```python
from build123d import *

# Parameters (mm, degrees)
SKETCH1_W                = 45
SKETCH1_H                = 40
BOSS_EXTRUDE1_DEPTH      = 50
SKETCH2_W                = 15
SKETCH2_H                = 10
CUT_EXTRUDE1_DEPTH       = 68.869359802
SKETCH6_W                = 20
SKETCH6_H                = 30
CUT_EXTRUDE15_DEPTH      = 33
CUT_EXTRUDE16_DEPTH      = 59.36308765
CUT_EXTRUDE16_DEPTH_BACK = 20


with BuildPart() as part:
    # Sketch1 → Boss-Extrude1 (new body)
    with BuildSketch(Plane(origin=(0, 0, 0), x_dir=(1, 0, 0), z_dir=(0, 1, 0))):
        Rectangle(SKETCH1_W, SKETCH1_H)
    extrude(amount=BOSS_EXTRUDE1_DEPTH)

    # Sketch2 → Cut-Extrude1 (cut, through all)
    with BuildSketch(Plane.XY.offset(20)):
        with Locations((0, 5)):
            Rectangle(SKETCH2_W, SKETCH2_H)
    extrude(amount=-CUT_EXTRUDE1_DEPTH, mode=Mode.SUBTRACT)

    # Sketch6 → Cut-Extrude15 (cut)
    with BuildSketch(Plane.ZY.offset(22.5)):
        with Locations((10, 35)):
            Rectangle(SKETCH6_W, SKETCH6_H)
    extrude(amount=-CUT_EXTRUDE15_DEPTH, mode=Mode.SUBTRACT)

    # Sketch7 → Cut-Extrude16 (cut, two sides: drawn at the far end of the back side and taken through both)
    with BuildSketch(Plane.XY.offset(-CUT_EXTRUDE16_DEPTH_BACK)):
        Polygon((106.556450077, 137.324045524), (10.5, 50), (-22.5, 20), (-118.556450077, -67.324045524), (-293.204541126, 124.788854629), (-68.091640972, 329.436945678), align=None)
    extrude(amount=CUT_EXTRUDE16_DEPTH + CUT_EXTRUDE16_DEPTH_BACK, mode=Mode.SUBTRACT)


solid = part.part
```
Geometry check sheet. Reference: the model listing, model coordinates, mm. A direction names the side the tool comes from. Coordinates: 2 decimals unless noted, no trailing zeros. Write each loop counter-clockwise with the first axis right and the second up, starting at its lowest first coordinate (ties: lowest second). Pieces come first, ordered by that corner, then holes. Notation, with made-up numbers: (-35, -33) -> (-13, -33) arc R21 ccw to (-13, 0) -> close; hole circle Ø11 at (-38.75, -23). An arc over 180 degrees is marked (long way). Use CSV: the item, a comma, the result in double quotes. Start each with the question number.
Item 1: Cross-section at A-A, the plane z = -10.5. Record the cut outline in (x, y), plus the area to 4 significant figures.
Item 2: Cross-section at B-B, the plane y = 39.5. Record the cut outline in (x, z), plus the area to 3 significant figures.
Item 3: Depth check by flat-ended pin: pin 1 Ø9 at (x, y) = (-11, 33) entering from +Z; pin 2 Ø2 at (x, z) = (-1.5, -9) entering from -Y; pin 3 Ø4 at (y, z) = (29.5, 13.5) entering from -X. Enter the tip coordinate at first touch or a pass-through.
Item 4: Thickness scan on line 1 (X direction, y = 4, z = -12.5); line 2 (X direction, y = 38, z = 15); line 3 (Z direction, x = 7.5, y = 42). Record the ranges inside material, lowest first.
Item 5: Mould release check, pull along X, two halves, no side actions. Record for faces 4 (the flat face through (22.5, 25, 0)), 5 (the flat face through (15, 0, 0)), 6 (the flat face through (0, 10, 0)): released by +X, released by -X, zero draft, split by the parting line, or undercut.
Item 6: Set-up check for faces 1 (the flat face through (5, 25, -20)), 2 (the flat face through (1, 28, 0)), 3 (the flat face through (7.5, 5, 0)): record each of +Z, -Z, +X, -X, +Y, -Y from which the full face is reachable in a straight line by a thin tool's end or side.
Item 7: Cross-section at D-D, the plane z = 10. Record the cut outline in (x, y).
Item 8: Cross-section at C-C, the plane x = -15. Record the cut outline in (y, z), plus the area to 3 significant figures.
Answers:
1,outline,"(-22.5, 0) -> (-7.5, 0) -> (-7.5, 10) -> (7.5, 10) -> (7.5, 0) -> (22.5, 0) -> (22.5, 50) -> (10.5, 50) -> (-22.5, 20) -> close"
1,area,"1,605 mm^2"
2,outline,"(-1.05, -20) -> (22.5, -20) -> (22.5, 20) -> (10.5, 20) -> (10.5, 0) -> (-1.05, 0) -> close"
2,area,"711 mm^2"
3,pin 1,"z = 0"
3,pin 2,"y = 10"
3,pin 3,"x = 10.5"
4,line 1,"-22.5 to -7.5, 7.5 to 22.5"
4,line 2,"10.5 to 22.5"
4,line 3,"-20 to 0"
5,face 4,"released by +X"
5,face 5,"zero draft"
5,face 6,"undercut"
6,face 1,"-Z, +X, -X, +Y, -Y"
6,face 2,"+Z, -X, +Y"
6,face 3,"+Z, -Z, -Y"
7,outline,"(-22.5, 0) -> (-7.5, 0) -> (-7.5, 10) -> (7.5, 10) -> (7.5, 0) -> (22.5, 0) -> (22.5, 50) -> (10.5, 50) -> (10.5, 20) -> (-22.5, 20) -> close"
8,outline,"(0, -20) -> (26.82, -20) -> (26.82, 0) -> (20, 0) -> (20, 20) -> (0, 20) -> close"
8,area,"936 mm^2"
